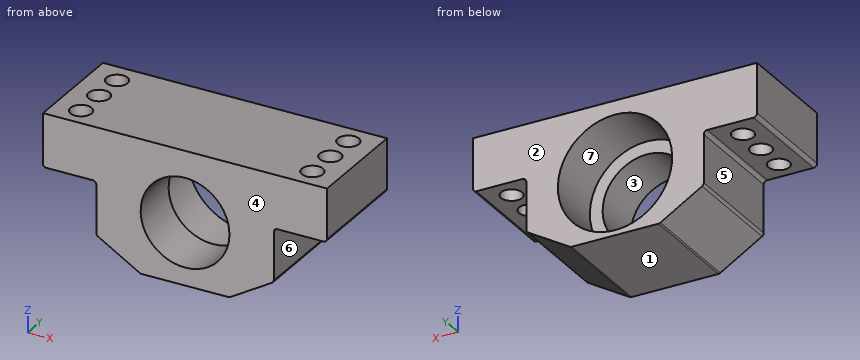
```python
from build123d import *

# Parameters (mm, degrees)
BOSS_EXTRUDE1_DEPTH = 30
SKETCH2_R           = 16.1
CUT_EXTRUDE1_DEPTH  = 16
SKETCH6_R           = 12.5
CUT_EXTRUDE2_DEPTH  = 14
SKETCH8_R           = 3
CUT_EXTRUDE4_DEPTH  = 15
SKETCH9_R           = 3
CUT_EXTRUDE5_DEPTH  = 15
CUT_EXTRUDE6_DEPTH  = 30
CUT_EXTRUDE7_DEPTH  = 30
CUT_EXTRUDE8_DEPTH  = 30
FILLET2_R           = 1
FILLET3_R           = 1


with BuildPart() as part:
    # Sketch1 → Boss-Extrude1 (new body)
    with BuildSketch(Plane(origin=(0, 0, 0), x_dir=(1, 0, 0), z_dir=(0, 1, 0))):
        Polygon((0, 0), (40, 0), (40, 15), (25, 15), (25, 45), (-25, 45), (-25, 15), (-40, 15), (-40, 0), align=None)
    extrude(amount=BOSS_EXTRUDE1_DEPTH)

    # Sketch2 → Cut-Extrude1 (cut)
    with BuildSketch(Plane(origin=(0, 30, 0), x_dir=(1, 0, 0), z_dir=(0, 1, 0))):
        with Locations(Location((0, 20, 0), (0, 0, 270))):
            Circle(SKETCH2_R)
    extrude(amount=-CUT_EXTRUDE1_DEPTH, mode=Mode.SUBTRACT)

    # Sketch6 → Cut-Extrude2 (cut)
    with BuildSketch(Plane.XZ):
        with Locations(Location((0, -20, 0), (0, 0, 270))):
            Circle(SKETCH6_R)
    extrude(amount=-CUT_EXTRUDE2_DEPTH, mode=Mode.SUBTRACT)

    # Sketch8 → Cut-Extrude4 (cut)
    with BuildSketch(Plane(origin=(0, 0, -15), x_dir=(-1, 0, 0), z_dir=(0, 0, -1))):
        with Locations((-32.5, 6)):
            Circle(SKETCH8_R)
        with Locations((-32.5, 15)):
            Circle(SKETCH8_R)
        with Locations((-32.5, 24)):
            Circle(SKETCH8_R)
    extrude(amount=-CUT_EXTRUDE4_DEPTH, mode=Mode.SUBTRACT)

    # Sketch9 → Cut-Extrude5 (cut)
    with BuildSketch(Plane(origin=(0, 0, -15), x_dir=(-1, 0, 0), z_dir=(0, 0, -1))):
        with Locations((32.5, 23.72166378)):
            Circle(SKETCH9_R)
        with Locations((32.5, 14.72166378)):
            Circle(SKETCH9_R)
        with Locations((32.5, 5.72166378)):
            Circle(SKETCH9_R)
    extrude(amount=-CUT_EXTRUDE5_DEPTH, mode=Mode.SUBTRACT)

    # Sketch11 → Cut-Extrude6 (cut)
    with BuildSketch(Plane(origin=(0, 30, 0), x_dir=(1, 0, 0), z_dir=(0, 1, 0))):
        Polygon((-25, 30), (-25, 45), (0, 45), align=None)
    extrude(amount=-CUT_EXTRUDE6_DEPTH, mode=Mode.SUBTRACT)

    # Sketch12 → Cut-Extrude7 (cut)
    with BuildSketch(Plane(origin=(0, 30, 0), x_dir=(1, 0, 0), z_dir=(0, 1, 0))):
        Polygon((25, 30), (0, 45), (25, 45), align=None)
    extrude(amount=-CUT_EXTRUDE7_DEPTH, mode=Mode.SUBTRACT)

    # Sketch13 → Cut-Extrude8 (cut)
    with BuildSketch(Plane(origin=(0, 30, 0), x_dir=(1, 0, 0), z_dir=(0, 1, 0))):
        Polygon((-12.5, 37.5), (12.5, 37.5), (0, 45), align=None)
    extrude(amount=-CUT_EXTRUDE8_DEPTH, mode=Mode.SUBTRACT)

    # Fillet2
    fillet2_edges = [part.edges().sort_by_distance(p)[0] for p in [
        (-25, 15, -15),
    ]]
    fillet(fillet2_edges, radius=FILLET2_R)

    # Fillet3
    fillet3_edges = [part.edges().sort_by_distance(p)[0] for p in [
        (-40, 15, -15),
        (25, 15, -15),
        (40, 15, -15),
        (-25, 15, -30),
        (25, 15, -30),
        (-12.5, 15, -37.5),
        (12.5, 15, -37.5),
    ]]
    fillet(fillet3_edges, radius=FILLET3_R)


solid = part.part
```
Input: part model. Units: mm. Frame: model coordinates. Face numbers are marked on the shaded views. A direction names the side the tool comes from. Give positions to 0.01 mm unless a question says otherwise; leave off trailing zeros. Loops run counter-clockwise (first coordinate to the right, second up) from the corner with the lowest first, then second, coordinate; pieces in that order, holes last.
1) Section query C-C on x = -32.5. Return the cut outline in (y, z), and give its area (3 significant figures).
A:
outline: (0, -15) - (2.72, -15) - (2.72, 0) - (0, 0) - close; (8.72, -15) - (11.72, -15) - (11.72, 0) - (8.72, 0) - close; (17.72, -15) - (20.72, -15) - (20.72, 0) - (17.72, 0) - close; (26.72, -15) - (30, -15) - (30, 0) - (26.72, 0) - close
area: 180 mm2
2) Line query: L1, parallel to Y at x = -32, z = -3; L2, parallel to X at y = 25.5, z = -14.5; L3, parallel to Y at x = 31, z = -13.5. Output: solid intervals per line, ascending.
A:
L1: y = 0 to 2.76, 8.68 to 11.76, 17.68 to 20.76, 26.68 to 30
L2: x = -39.87 to -34.92, -30.08 to -15.13, 15.13 to 29.9, 35.1 to 39.87
L3: y = 0 to 3.4, 8.6 to 12.4, 17.6 to 21.4, 26.6 to 30
3) Section query A-A on y = 10.75. Return the cut outline in (x, z).
A:
outline: (-40, -14) arc R1 ccw to (-39, -15) - (-26, -15) arc R1 cw to (-25, -16) - (-25, -29.43) arc R1 ccw to (-24.51, -30.29) - (-12.74, -37.36) arc R1 ccw to (-12.22, -37.5) - (12.22, -37.5) arc R1 ccw to (12.74, -37.36) - (24.51, -30.29) arc R1 ccw to (25, -29.43) - (25, -16) arc R1 cw to (26, -15) - (39, -15) arc R1 ccw to (40, -14) - (40, 0) - (-40, 0) - close; hole circle Ø25 at (0, -20)
4) Section query B-B on z = -20. Return the cut outline in (x, y), and give its area (3 significant figures).
A:
outline: (-25, 0) - (-12.5, 0) - (-12.5, 14) - (-16.1, 14) - (-16.1, 30) - (-25, 30) - close; (12.5, 0) - (25, 0) - (25, 30) - (16.1, 30) - (16.1, 14) - (12.5, 14) - close
area: 635 mm2
5) Section query D-D on y = 25. Return the cut outline in (x, z).
A:
outline: (-40, -14) arc R1 ccw to (-39, -15) - (-35.21, -15) - (-35.21, 0) - (-40, 0) - close; (-29.79, -15) - (-26, -15) arc R1 cw to (-25, -16) - (-25, -29.43) arc R1 ccw to (-24.51, -30.29) - (-12.74, -37.36) arc R1 ccw to (-12.22, -37.5) - (12.22, -37.5) arc R1 ccw to (12.74, -37.36) - (24.51, -30.29) arc R1 ccw to (25, -29.43) - (25, -16) arc R1 cw to (26, -15) - (29.67, -15) - (29.67, 0) - (-29.79, 0) - close; (35.33, -15) - (39, -15) arc R1 ccw to (40, -14) - (40, 0) - (35.33, 0) - close; hole circle Ø32.2 at (0, -20)
6) Reachability of the marked faces 4, 5, 6 and 7 from +Z, -Z, +X, -X, +Y, -Y: full face, straight path, thin tool, end or side. Return the list, or none.
A:
face 4: +Z, -Z, +X, -X, -Y
face 5: -Z, -X, +Y, -Y
face 6: -Z, +X, +Y, -Y
face 7: +Y
7) Mould query, pull axis Z, two halves, no side actions, for the marked faces 1, 2 and 3. Classes: released by +Z, released by -Z, zero draft, split by the parting line, or undercut.
A:
face 1: released by -Z
face 2: zero draft
face 3: undercut
8) Contact query for flat-ended pins moving along their axis: pin 1 (3.5 mm diameter, centred on x = -32.5, y = 5.72, fed in from -Z); pin 2 (1 mm diameter, centred on y = 8, z = -26, fed in from -X); pin 3 (10.5 mm diameter, centred on x = -30.5, y = 10.5, fed in from -Z); pin 4 (4 mm diameter, centred on y = 22, z = -23, fed in from +X). Output: stop coordinate, or through.
A:
pin 1: passes through
pin 2: stops at x = -25
pin 3: stops at z = -15.34
pin 4: stops at x = 25
